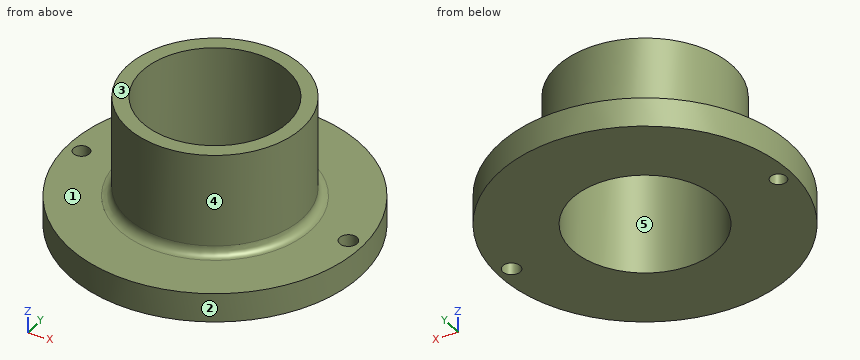
```python
from build123d import *

# Parameters (mm, degrees)
SKETCH1_R           = 50
SKETCH1_R_2         = 25
BOSS_EXTRUDE1_DEPTH = 10
SKETCH2_R           = 30
SKETCH2_R_2         = 25
BOSS_EXTRUDE2_DEPTH = 45
FILLET1_R           = 3
SKETCH3_R           = 3
SKETCH3_R_2         = 2.728941423
CUT_EXTRUDE1_DEPTH  = 50


with BuildPart() as part:
    # Sketch1 → Boss-Extrude1 (new body)
    with BuildSketch(Plane.XY):
        Circle(SKETCH1_R)
        Circle(SKETCH1_R_2, mode=Mode.SUBTRACT)
    extrude(amount=BOSS_EXTRUDE1_DEPTH)

    # Sketch2 → Boss-Extrude2 (add)
    with BuildSketch(Plane.XY):
        Circle(SKETCH2_R)
        Circle(SKETCH2_R_2, mode=Mode.SUBTRACT)
    extrude(amount=BOSS_EXTRUDE2_DEPTH)

    # Fillet1
    fillet1_edges = [part.edges().sort_by_distance(p)[0] for p in [
        (-30, 0, 10),
    ]]
    fillet(fillet1_edges, radius=FILLET1_R)

    # Sketch3 → Cut-Extrude1 (cut)
    with BuildSketch(Plane.XY):
        with Locations((45.016491683, 0)):
            Circle(SKETCH3_R)
        with Locations((-45.016491683, 0)):
            Circle(SKETCH3_R_2)
    extrude(amount=CUT_EXTRUDE1_DEPTH, mode=Mode.SUBTRACT)


solid = part.part
```
CAD build for the part. Positions are in the model's coordinates, mm. Face numbers are marked on the shaded views. A direction names the side the tool comes from. Round coordinates to 2 decimals unless told otherwise and drop trailing zeros. Order: outer loops, then holes, each group sorted by start corner. A loop starts at its lowest first (then second) coordinate and runs counter-clockwise, first axis right, second up. Notation, with made-up numbers: (34, 3) - (89, 3) arc R21 cw to (89, 8) - close; hole circle Ø9 at (70, 49.25). An arc over 180 degrees is marked (long way). Answer as CSV lines item,"result". Start each with the question number.
1. Saw through at D-D, the plane z = 18. Write the cut outline in (x, y).
2. Saw through at C-C, the plane z = 7. Write the cut outline in (x, y), and give its area (3 significant figures).
3. Drill centre lines: L1, parallel to Y at x = 0, z = 28; L2, parallel to Z at x = -36, y = 6; L3, parallel to X at y = 17.5, z = 29. Where is each one in solid material? Low to high. Write a range as [from, to].
4. Saw through at B-B, the plane y = 0. Write the cut outline in (x, z), and give its area (3 significant figures).
5. Tool access for the marked faces 1 and 2: list every direction of +Z, -Z, +X, -X, +Y, -Y with a clear straight run to the whole face (end or side of a thin tool).
6. Pin check, flat tips, straight feed: pin 1 (8 mm diameter, centred on y = -21, z = 32, fed in from +X); pin 2 (8 mm diameter, centred on x = -27.5, z = 39.5, fed in from +Y); pin 3 (3 mm diameter, centred on x = 4.5, z = 13, fed in from -Y). Stop position of each tip, or through.
7. Pull direction X, two halves, no side cores. Call the marked faces 3, 4 and 5: +X half, -X half, draft (parallel to the pull), parting line (faces both ways), or undercut.
8. Saw through at A-A, the plane x = 0. Write the cut outline in (y, z).
Model answer:
1,outline,"circle Ø60 at (0, 0); hole circle Ø50 at (0, 0)"
2,outline,"circle Ø100 at (0, 0); hole circle Ø5.46 at (-45.02, 0); hole circle Ø50 at (0, 0); hole circle Ø6 at (45.02, 0)"
2,area,"5,840 mm²"
3,L1,"y = [-30, -25], [25, 30]"
3,L2,"z = [0, 10]"
3,L3,"x = [-24.37, -17.85], [17.85, 24.37]"
4,outline,"(-50, 0) - (-47.75, 0) - (-47.75, 10) - (-50, 10) - close; (-42.29, 0) - (-25, 0) - (-25, 45) - (-30, 45) - (-30, 13) arc R3 cw to (-33, 10) - (-42.29, 10) - close; (25, 0) - (42.02, 0) - (42.02, 10) - (33, 10) arc R3 cw to (30, 13) - (30, 45) - (25, 45) - close; (48.02, 0) - (50, 0) - (50, 10) - (48.02, 10) - close"
4,area,"739 mm²"
5,face 1,"+Z"
5,face 2,"+Z, -Z"
6,pin 1,"stops at x = 24.72"
6,pin 2,"stops at y = 18.65"
6,pin 3,"stops at y = -30.09"
7,face 3,"draft"
7,face 4,"parting line"
7,face 5,"undercut"
8,outline,"(-50, 0) - (-25, 0) - (-25, 45) - (-30, 45) - (-30, 13) arc R3 cw to (-33, 10) - (-50, 10) - close; (25, 0) - (50, 0) - (50, 10) - (33, 10) arc R3 cw to (30, 13) - (30, 45) - (25, 45) - close"
